Build history of the part. All positions in model axes, mm. A direction names the side the tool comes from. Round coordinates to 2 decimals unless told otherwise and drop trailing zeros. Write each loop counter-clockwise with the first axis right and the second up, starting at its lowest first coordinate (ties: lowest second). Pieces come first, ordered by that corner, then holes. Notation, with made-up numbers: M -19.75,15.25 L 39.25,15.25 A21 cw 39.25,25.25 Z; hole C 10,2.5 d4. An arc over 180 degrees is marked long. Write item = value, one per line.
Autodesk Fusion 360 part; units mm, degrees
sketch "Sketch1" plane through (0, 0, 0) normal (0, 0, 1) x (1, 0, 0)
  line L0 (0, 0) -> (300, 0)
  line L1 (300, 0) -> (300, 1200)
  line L2 (300, 1200) -> (0, 1200)
  line L3 (0, 600) -> (-300, 600)
  line L4 (-300, 600) -> (-300, 1800)
  line L5 (-300, 1800) -> (0, 1800)
  line L6 (0, 1800) -> (0, 1200)
  line L7 (0, 0) -> (0, 600)
  line L8 (20, 1820) -> (20, 1220)
  line L9 (320, 1220) -> (20, 1220)
  line L10 (320, -20) -> (320, 1220)
  line L11 (-20, -20) -> (320, -20)
  line L12 (-20, -20) -> (-20, 580)
  line L13 (-20, 580) -> (-320, 580)
  line L14 (-320, 580) -> (-320, 1820)
  line L15 (-320, 1820) -> (20, 1820)
  dimension "d1" = 300
  dimension "d2" = 1200
  dimension "d3" = 300
  dimension "d4" = 1200
  dimension "d5" = -20
extrude "Extrude1" add sketch "Sketch1" along normal blind 400 makes body 1
extrude "Extrude2" add sketch "Sketch1" against normal blind 5 separate body contours L0 L1 L2 L3 L4 L5 L6 L7 makes body 2
extrude "Extrude3" add sketch "Sketch1" against normal blind 5 bodies 1 2
extrude "Extrude4" cut 1 faces at (-313.3333, 1400, 400) along direction (0, 0, -1) blind 100 on bodies 1 bodies 1
extrude "Extrude5" cut 1 faces at (-313.3333, 1400, 300) along direction (0, 0, -1) blind 50 on bodies 1 bodies 1
sketch "Sketch2" plane through (300, 0, 0) normal (-1, 0, 0) x (0, -1, 0)
  line L0 (0, 250) -> (-1200, 250)
  line L1 (-1200, 250) -> (-1200, 0)
  line L2 (-1200, 0) -> (0, 0)
  line L3 (0, 0) -> (0, 250)
  line L4 (-600, 250) -> (-600, 0) construction
  line L5 (-1200, 250) -> (-1200, 200) construction
  line L6 (-1200, 200) -> (-600, 0)
  dimension "d16" = 50
extrude "Extrude6" add sketch "Sketch2" along normal blind 300 contours L1 L2 L6 bodies 1
sketch "Sketch3" plane through (-300, 0, 0) normal (1, 0, 0) x (0, 1, 0)
  line L0 (1800, 250) -> (600, 250)
  line L1 (600, 250) -> (600, 0)
  line L2 (600, 0) -> (1800, 0)
  line L3 (1800, 0) -> (1800, 250)
  line L4 (1200, 250) -> (1200, 0) construction
  line L5 (600, 250) -> (600, 200) construction
  line L6 (600, 200) -> (1200, 0)
  dimension "d19" = 50
extrude "Extrude7" add sketch "Sketch3" along normal blind 300 contours L1 L2 L6 bodies 1
sketch "Sketch4" plane through (0, 0, 0) normal (-1, 0, 0) x (0, -1, 0)
  line L0 (-1200, 0) -> (-900, 100)
  line L1 (-900, 100) -> (-1200, 200)
  line L2 (-1200, 200) -> (-1200, 250)
  line L3 (-1200, 250) -> (-1800, 250)
  line L4 (-1800, 250) -> (-1800, 0)
  line L5 (-1800, 0) -> (-1200, 0)
  line L6 (-900, 100) -> (-900, 150)
  line L7 (-1200, 250) -> (-900, 150)
  dimension "d22" = 50
sketch "Sketch5" plane through (0, 0, 0) normal (1, 0, 0) x (0, 1, 0)
  line L0 (600, 250) -> (0, 250)
  line L1 (0, 250) -> (0, 0)
  line L2 (0, 0) -> (600, 0)
  line L3 (600, 0) -> (900, 100)
  line L4 (900, 100) -> (600, 200)
  line L5 (600, 200) -> (600, 250)
  line L6 (900, 100) -> (900, 150)
  line L7 (900, 150) -> (600, 250)
  dimension "d23" = 50
extrude "Extrude8" add sketch "Sketch5" sketch "Sketch4" against normal mid plane 20 contours L4 L5 L6 L7 of sketch 2 contours L1 L2 L6 L7 bodies 1
sketch "Sketch6" plane through (0, 0, 0) normal (-1, 0, 0) x (0, -1, 0)
  line L0 (-1200, 0) -> (-900, 100)
  line L1 (-900, 100) -> (-1200, 200)
  line L2 (-1200, 200) -> (-1200, 250)
  line L3 (-1200, 250) -> (-1800, 250)
  line L4 (-1800, 250) -> (-1800, 0)
  line L5 (-1800, 0) -> (-1200, 0)
  line L6 (-1200, 0) -> (-1200, 200)
extrude "Extrude9" add sketch "Sketch6" along normal blind 10 contours L0 L1 L6 bodies 1
sketch "Sketch7" plane through (0, 0, 0) normal (1, 0, 0) x (0, 1, 0)
  line L0 (600, 250) -> (0, 250)
  line L1 (0, 250) -> (0, 0)
  line L2 (0, 0) -> (600, 0)
  line L3 (600, 0) -> (900, 100)
  line L4 (900, 100) -> (600, 200)
  line L5 (600, 200) -> (600, 250)
  line L6 (600, 200) -> (600, 0)
extrude "Extrude10" add sketch "Sketch7" along normal blind 10 contours L3 L4 L6 bodies 1
1. Band-saw the part on C-C (y = 293.5). List the corners of the cut face in (x, z).
Responses:
outline = M -20,-5 L 320,-5 L 320,250 L 300,250 L 300,0 L 0,0 L 0,250 L -20,250 Z
2. Flat gauge pins, fed straight in: pin 1 (8 mm diameter, centred on x = -116, z = 52, fed in from -Y); pin 2 (5 mm diameter, centred on x = -25, y = 1053, fed in from +Z); pin 3 (6 mm diameter, centred on x = 157.5, z = 108, fed in from +Y). Where does each tip first touch, or does it go through?
Responses:
pin_1 = 580
pin_2 = 49.83
pin_3 = 1220
3. Probe probe 1 along X at (y, z) = (652.5, 98); probe 2 along Y at (x, z) = (-80, 202); probe 3 along X at (y, z) = (1178.5, 67). List the from-to ranges inside material, lowest first.
Responses:
probe_1 = -320 to 10, 300 to 320
probe_2 = 580 to 600, 1800 to 1820
probe_3 = -320 to -300, -10 to 320
4. Tool access for faces 1 (the face through (-157, 895.8, 101.4)), 2 (the face through (-168, 580, 121)), 3 (the face through (320, 591, 121)): list every direction of +Z, -Z, +X, -X, +Y, -Y with a clear straight run to the whole face (end or side of a thin tool).
Responses:
face_1 = +Z
face_2 = +Z, -Z, -X, -Y
face_3 = +Z, -Z, +X, +Y, -Y
5. Mould opens along Y. For faces 4 (the face through (-1, 564, 250)), 5 (the face through (0.1, 752.1, 199.3)), 6 (the face through (-152, 1820, 121)) say: pulls with the +Y half, pulls with the -Y half, needs draft (parallel to the pull), parting line crosses it, or undercut.
Responses:
face_4 = needs draft
face_5 = undercut
face_6 = pulls with the +Y half
6. Band-saw the part on D-D (x = 100). List the corners of the cut face in (y, z).
Responses:
outline = M -20,-5 L 1220,-5 L 1220,250 L 1200,250 L 1200,200 L 600,0 L 0,0 L 0,250 L -20,250 Z
7. Band-saw the part on A-A (z = 118). List the corners of the cut face in (x, y), plus the area to 3 significant figures.
Responses:
outline = M -320,580 L -20,580 L -20,-20 L 320,-20 L 320,1220 L 20,1220 L 20,1820 L -320,1820 Z; hole M -300,846 L -10,846 L -10,1200 L 0,1200 L 0,1800 L -300,1800 Z; hole M 0,0 L 300,0 L 300,954 L 10,954 L 10,600 L 0,600 Z
area = 252,000 mm²
8. Band-saw the part on B-B (z = 232). List the corners of the cut face in (x, y).
Responses:
outline = M -320,580 L -20,580 L -20,-20 L 320,-20 L 320,1220 L 20,1220 L 20,1820 L -320,1820 Z; hole M -300,600 L -10,600 L -10,654 L 10,654 L 10,600 L 0,600 L 0,0 L 300,0 L 300,1200 L 10,1200 L 10,1146 L -10,1146 L -10,1200 L 0,1200 L 0,1800 L -300,1800 Z
